Geometry: final body of the model. Coordinates: model frame, mm. Face numbers are marked on the shaded views. A direction names the side the tool comes from. Give positions to 0.01 mm unless a question says otherwise; leave off trailing zeros. Write each loop counter-clockwise with the first axis right and the second up, starting at its lowest first coordinate (ties: lowest second). Pieces come first, ordered by that corner, then holes. Notation, with made-up numbers: (-32, 69.5) -> (22, 69.5) arc R33 ccw to (22, 98.5) -> close; hole circle Ø8 at (62, -16.5). An arc over 180 degrees is marked (long way). Answer as a JSON object with one key per item and string values.
from build123d import *

# Parameters (mm, degrees)
SKETCH2_W           = 74
SKETCH2_H           = 62
BOSS_EXTRUDE1_DEPTH = 10
BOSS_EXTRUDE2_DEPTH = 11
SKETCH5_R           = 4.25
CUT_EXTRUDE2_DEPTH  = 75
FILLET1_R           = 2


with BuildPart() as part:
    # Sketch2 → Boss-Extrude1 (new body)
    with BuildSketch(Plane(origin=(0, 0, 0), x_dir=(1, 0, 0), z_dir=(0, 1, 0))):
        with Locations((37, 31)):
            Rectangle(SKETCH2_W, SKETCH2_H)
    extrude(amount=BOSS_EXTRUDE1_DEPTH)

    # Sketch3 → Boss-Extrude2 (add)
    with BuildSketch(Plane.XY):
        with BuildLine():
            Line((22, 10), (22, 38))
            ThreePointArc((22, 38), (37, 53), (52, 38))
            Line((52, 38), (52, 10))
            Line((52, 10), (22, 10))
        make_face()
    boss_extrude2 = extrude(amount=-BOSS_EXTRUDE2_DEPTH)

    # Mirror1: Boss-Extrude2 across plane
    add(boss_extrude2.mirror(Plane.XY.offset(-31)))

    # Sketch5 → Cut-Extrude2 (cut)
    with BuildSketch(Plane(origin=(0, 0, -62), x_dir=(-1, 0, 0), z_dir=(0, 0, -1))):
        with Locations((-37, 38)):
            Circle(SKETCH5_R)
    extrude(amount=-CUT_EXTRUDE2_DEPTH, mode=Mode.SUBTRACT)

    # Fillet1
    fillet1_edges = [part.edges().sort_by_distance(p)[0] for p in [
        (74, 10, -31),
        (63, 10, -62),
        (63, 10, 0),
        (37, 10, -11),
        (52, 10, -5.5),
        (22, 24, -11),
        (22, 10, -5.5),
        (37, 53, -11),
        (52, 24, -11),
        (52, 24, 0),
        (37, 53, 0),
        (22, 24, 0),
        (11, 10, -62),
        (22, 10, -56.5),
        (52, 24, -62),
        (52, 10, -56.5),
        (37, 53, -62),
        (0, 10, -31),
        (22, 24, -62),
        (37, 10, -51),
        (52, 24, -51),
        (37, 53, -51),
        (22, 24, -51),
        (11, 10, 0),
    ]]
    fillet(fillet1_edges, radius=FILLET1_R)


solid = part.part
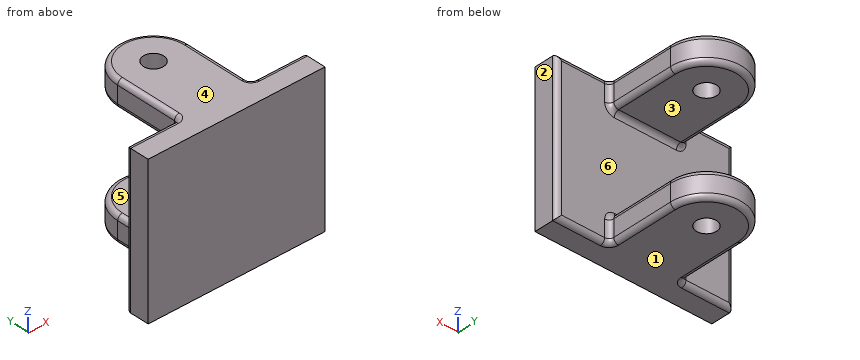
Q1. Material intervals for L1, parallel to Z at x = 24.5, y = 37.5; L2, parallel to Y at x = 37, z = -8; L3, parallel to Y at x = 5.5, z = -53, sorted ascending. Write a range as from..to.
Values:
{"L1": "-62..-51, -11..0", "L2": "0..33.75, 42.25..53", "L3": "0..10"}
Q2. First-contact query: P1, Ø7.5, axis at y = 20, z = -4.5, coming from the -X side; P2, Ø3.5, axis at y = 29.5, z = -55, coming from the +X side; P3, Ø6, axis at x = 22.5, z = -19.5, coming from the +Y side. Flat tips, straight axial feed; report the tip coordinate or a pass-through.
Values:
{"P1": "x = 22", "P2": "x = 52", "P3": "y = 10"}
Q3. Cut plane C-C (z = -30.5). Return the cut outline in (x, y), and give its area (3 significant figures).
Values:
{"outline": "(0, 0) -> (74, 0) -> (74, 8) arc R2 ccw to (72, 10) -> (2, 10) arc R2 ccw to (0, 8) -> close", "area": "738 mm²"}
Q4. Cut plane A-A (x = 37). Return the cut outline in (y, z), and give its area (3 significant figures).
Values:
{"outline": "(0, -62) -> (33.75, -62) -> (33.75, -51) -> (12, -51) arc R2 cw to (10, -49) -> (10, -13) arc R2 cw to (12, -11) -> (33.75, -11) -> (33.75, 0) -> (0, 0) -> close; (42.25, -62) -> (51, -62) arc R2 ccw to (53, -60) -> (53, -53) arc R2 ccw to (51, -51) -> (42.25, -51) -> close; (42.25, -11) -> (51, -11) arc R2 ccw to (53, -9) -> (53, -2) arc R2 ccw to (51, 0) -> (42.25, 0) -> close", "area": "1,380 mm²"}
Q5. Cut plane D-D (y = 35.5). Return the cut outline in (x, z), and give its area (3 significant figures).
Values:
{"outline": "(22, -60) arc R2 ccw to (24, -62) -> (33.56, -62) -> (33.56, -51) -> (24, -51) arc R2 ccw to (22, -53) -> close; (22, -9) arc R2 ccw to (24, -11) -> (33.56, -11) -> (33.56, 0) -> (24, 0) arc R2 ccw to (22, -2) -> close; (40.44, -62) -> (50, -62) arc R2 ccw to (52, -60) -> (52, -53) arc R2 ccw to (50, -51) -> (40.44, -51) -> close; (40.44, -11) -> (50, -11) arc R2 ccw to (52, -9) -> (52, -2) arc R2 ccw to (50, 0) -> (40.44, 0) -> close", "area": "502 mm²"}
Q6. Mould query, pull axis Z, two halves, no side actions, for the marked faces 1, 2 and 3. Classes: pulls with the +Z half, pulls with the -Z half, needs draft (parallel to the pull), parting line crosses it, or undercut.
Values:
{"face 1": "pulls with the -Z half", "face 2": "needs draft", "face 3": "undercut"}
Q7. Cut plane B-B (y = 18). Return the cut outline in (x, z).
Values:
{"outline": "(22, -60) arc R2 ccw to (24, -62) -> (50, -62) arc R2 ccw to (52, -60) -> (52, -53) arc R2 ccw to (50, -51) -> (24, -51) arc R2 ccw to (22, -53) -> close; (22, -9) arc R2 ccw to (24, -11) -> (50, -11) arc R2 ccw to (52, -9) -> (52, -2) arc R2 ccw to (50, 0) -> (24, 0) arc R2 ccw to (22, -2) -> close"}
Q8. Set-up query: the marked faces 4, 5 and 6. Return all of +Z, -Z, +X, -X, +Y, -Y with unobstructed straight access to the full face (end or side cutting, diameter ignored); none if empty.
Values:
{"face 4": "+Z, +X, -X, +Y, -Y", "face 5": "+X, -X, +Y", "face 6": "+Y"}
